```python
from build123d import *

# Parameters (mm, degrees)
SKETCH1_R           = 35
SKETCH1_R_2         = 12.8
BOSS_EXTRUDE1_DEPTH = 31
SKETCH4_R           = 25.97
CUT_EXTRUDE3_DEPTH  = 19
SKETCH10_R          = 2.125
CUT_EXTRUDE6_DEPTH  = 5.1


with BuildPart() as part:
    # Sketch1 → Boss-Extrude1 (new body)
    with BuildSketch(Plane(origin=(0, 0, 0), x_dir=(1, 0, 0), z_dir=(0, 1, 0))):
        with Locations(Location((0, 0, 0), (0, 0, 270))):
            Circle(SKETCH1_R)
        with Locations(Location((0, 0, 0), (0, 0, 270))):
            Circle(SKETCH1_R_2, mode=Mode.SUBTRACT)
    extrude(amount=BOSS_EXTRUDE1_DEPTH)

    # Sketch4 → Cut-Extrude3 (cut)
    with BuildSketch(Plane(origin=(0, 31, 0), x_dir=(1, 0, 0), z_dir=(0, 1, 0))):
        with Locations(Location((0, 0, 0), (0, 0, 270))):
            Circle(SKETCH4_R)
    extrude(amount=-CUT_EXTRUDE3_DEPTH, mode=Mode.SUBTRACT)

    # Sketch10 → Cut-Extrude6 (cut)
    with BuildSketch(Plane.XZ):
        with Locations(Location((-25.362762045, -1.374882343, 0), (0, 0, 270))):
            Circle(SKETCH10_R)
        with Locations(Location((11.490697986, 22.652237412, 0), (0, 0, 270))):
            Circle(SKETCH10_R)
        with Locations(Location((13.872064059, -21.277355069, 0), (0, 0, 270))):
            Circle(SKETCH10_R)
    extrude(amount=-CUT_EXTRUDE6_DEPTH, mode=Mode.SUBTRACT)


solid = part.part
```
Design review of the part built by this model. Coordinates are the model's own, in mm. A direction names the side the tool comes from. Give positions to 0.01 mm unless a question says otherwise; leave off trailing zeros. Write each loop counter-clockwise with the first axis right and the second up, starting at its lowest first coordinate (ties: lowest second). Pieces come first, ordered by that corner, then holes.
(1) Add section B-B (y = 17.5). Give the boundary of the cut face in (x, z), and give its area (3 significant figures).
Checked values:
outline: circle Ø70 at (0, 0); hole circle Ø51.94 at (0, 0)
area: 1,730 mm2
(2) Add section C-C (z = 17.5). Give the boundary of the cut face in (x, y).
Checked values:
outline: (-30.31, 0) - (30.31, 0) - (30.31, 31) - (19.19, 31) - (19.19, 12) - (-19.19, 12) - (-19.19, 31) - (-30.31, 31) - close
(3) Add section A-A (x = 0). Give the boundary of the cut face in (y, z), and give its area (3 significant figures).
Checked values:
outline: (0, -35) - (31, -35) - (31, -25.97) - (12, -25.97) - (12, -12.8) - (0, -12.8) - close; (0, 12.8) - (12, 12.8) - (12, 25.97) - (31, 25.97) - (31, 35) - (0, 35) - close
area: 876 mm2
(4) Wall thickness on line 1 along Z through (x, y) = (10.5, 5); line 2 along Y through (x, z) = (-17, 4); line 3 along Z through (x, y) = (-3, 24): over which ranges is each line inside the solid? List them lowest first.
Checked values:
line 1: z = -33.39 to -7.32, 7.32 to 20.77, 24.53 to 33.39
line 2: y = 0 to 12
line 3: z = -34.87 to -25.8, 25.8 to 34.87
(5) Add section D-D (x = 18). Give the boundary of the cut face in (y, z).
Checked values:
outline: (0, -30.02) - (31, -30.02) - (31, -18.72) - (12, -18.72) - (12, 18.72) - (31, 18.72) - (31, 30.02) - (0, 30.02) - close
(6) Mouldability with a two-part tool opening along Z and no side actions: class faces 1 (the face through (-15, 0, 0)), 2 (the face through (12, 5.1, 23)), 3 (the face through (-21, 15, -28)) as +Z half, -Z half, draft (parallel to the pull), parting line (faces both ways), or undercut.
Checked values:
face 1: draft
face 2: undercut
face 3: parting line
(7) Tool access review of faces 4 (the face through (-2.4, 31, -26.1)), 5 (the face through (7.8, 21.63, 24.77)), 6 (the face through (13.06, 2.51, -23.24)): name each direction out of +Z, -Z, +X, -X, +Y, -Y from which nothing blocks a thin tool from reaching the whole face with its end or side.
Checked values:
face 4: +Z, -Z, +X, -X, +Y
face 5: +Y
face 6: -Y
(8) Clearance check with flat-ended pins moving along their axes: pin 1 Ø3 at (x, z) = (-11, 5) entering from -Y; pin 2 Ø1 at (x, y) = (-20, 15) entering from -Z; pin 3 Ø3 at (y, z) = (17.5, 4) entering from -X; pin 4 Ø2 at (y, z) = (5.5, 8.5) entering from +X. State where each tip first meets the part, or that it passes through.
Checked values:
pin 1: stops at y = 0
pin 2: stops at z = -29.06
pin 3: stops at x = -34.91
pin 4: stops at x = 34.19
